Design review of the part built by this model. Coordinates are the model's own, in mm. A direction names the side the tool comes from. Give positions to 0.01 mm unless a question says otherwise; leave off trailing zeros. Loops run counter-clockwise (first coordinate to the right, second up) from the corner with the lowest first, then second, coordinate; pieces in that order, holes last. Notation, with made-up numbers: (-14.5, -11.5) - (28.5, -11.5) arc R11 cw to (28.5, -1.5) - close; hole circle Ø8 at (-1.5, -18.5). An arc over 180 degrees is marked (long way). Write each question's results on one line, items separated by ' | '.
```python
from build123d import *

# Parameters (mm, degrees)
SKETCH1_R                = 12.5
BOSS_EXTRUDE1_DEPTH      = 1.5
BOSS_EXTRUDE2_DEPTH      = 1.4
BOSS_EXTRUDE2_DEPTH_BACK = 1.4
SKETCH1_3_R              = 12.5
BODY_MOVE_COPY1_ANGLE    = 90


with BuildPart() as part:
    # Sketch1 → Boss-Extrude1 (new, symmetric)
    with BuildSketch(Plane(origin=(0, 0, 0), x_dir=(1, 0, 0), z_dir=(0, 1, 0))):
        with BuildLine():
            Line((-120, 35), (-120, -35))
            ThreePointArc((-120, -35), (-65.786340219, -20.263519795), (-10.172182489, -28.222804669))
            ThreePointArc((-10.172182489, -28.222804669), (30, 0), (-10.172182489, 28.222804669))
            ThreePointArc((-10.172182489, 28.222804669), (-65.786340219, 20.263519795), (-120, 35))
        make_face()
        with Locations(Location((0, 0, 0), (0, 0, 270))):
            Circle(SKETCH1_R, mode=Mode.SUBTRACT)
    extrude(amount=BOSS_EXTRUDE1_DEPTH, both=True)

    # Sketch1<3> → Boss-Extrude2 (add, two sides: drawn at the far end of the back side and taken through both)
    with BuildSketch(Plane(origin=(0, 0, 0), x_dir=(1, 0, 0), z_dir=(0, 1, 0)).offset(-BOSS_EXTRUDE2_DEPTH_BACK)):
        with Locations(Location((0, 0, 0), (0, 0, 90))):
            Circle(SKETCH1_3_R)
    extrude(amount=BOSS_EXTRUDE2_DEPTH + BOSS_EXTRUDE2_DEPTH_BACK)


with BuildPart() as part_1:
    # Body-Move/Copy1: moved
    add(part.part.rotate(Axis((0, 0, 0), (1, 0, 0)), BODY_MOVE_COPY1_ANGLE))


solid = part_1.part
```
Item 1: We need section B-B on x = 0. Give the boundary of the cut face in (y, z).
Output values:
outline: (-30, -1.5) - (-12.5, -1.5) - (-12.5, -1.4) - (12.5, -1.4) - (12.5, -1.5) - (30, -1.5) - (30, 1.5) - (12.5, 1.5) - (12.5, 1.4) - (-12.5, 1.4) - (-12.5, 1.5) - (-30, 1.5) - close
Item 2: We need section D-D on z = 0. Give the boundary of the cut face in (x, y), then the cut area to 3 significant figures.
Output values:
outline: (-120, -35) arc R138.81 cw to (-10.17, -28.22) arc R30 ccw (long way) to (-10.17, 28.22) arc R138.81 cw to (-120, 35) - close | area: 7,270 mm²
Item 3: We need section A-A on y = -24.5. Give the boundary of the cut face in (x, z).
Output values:
outline: (-120, -1.5) - (-92.29, -1.5) - (-92.29, 1.5) - (-120, 1.5) - close; (-22.18, -1.5) - (17.31, -1.5) - (17.31, 1.5) - (-22.18, 1.5) - close
Item 4: Tool access review of faces 5 (the face through (-46, 0, -1.5)), 6 (the face through (0, 0, 1.4)), 7 (the face through (0, 0, -1.4)): name each direction out of +Z, -Z, +X, -X, +Y, -Y from which nothing blocks a thin tool from reaching the whole face with its end or side.
Output values:
face 5: -Z, +X, -X, +Y, -Y | face 6: +Z | face 7: -Z
Item 5: Draft analysis for pull direction X (two halves, no side actions). For faces 1 (the face through (-46, 0, 1.5)), 2 (the face through (-66.577, -20.315, 0.021)), 3 (the face through (-120, 0, 0)), 4 (the face through (29.99, -0.8, 0.02)), state which applies: +X half, -X half, draft (parallel to the pull), parting line (faces both ways), or undercut.
Output values:
face 1: draft | face 2: undercut | face 3: -X half | face 4: undercut
Item 6: Clearance check with a flat-ended pin moving along its axis: P1, Ø1.5, axis at x = -97, z = 0, coming from the -Y side. State where the tip first meets the part, or that it passes through.
Output values:
P1: stops at y = -26.04
Item 7: Wall thickness on probe 1 along Y at (x, z) = (-1, -0.55); probe 2 along Z at (x, y) = (-5.5, -7); probe 3 along Y at (x, z) = (-5, -1.1): over which ranges is each line inside the solid? List them lowest first.
Output values:
probe 1: y = -29.98 to 29.98 | probe 2: z = -1.4 to 1.4 | probe 3: y = -29.58 to 29.58
Item 8: We need section C-C on y = 26. Give the boundary of the cut face in (x, z).
Output values:
outline: (-120, -1.5) - (-97.61, -1.5) - (-97.61, 1.5) - (-120, 1.5) - close; (-16.87, -1.5) - (14.97, -1.5) - (14.97, 1.5) - (-16.87, 1.5) - close
